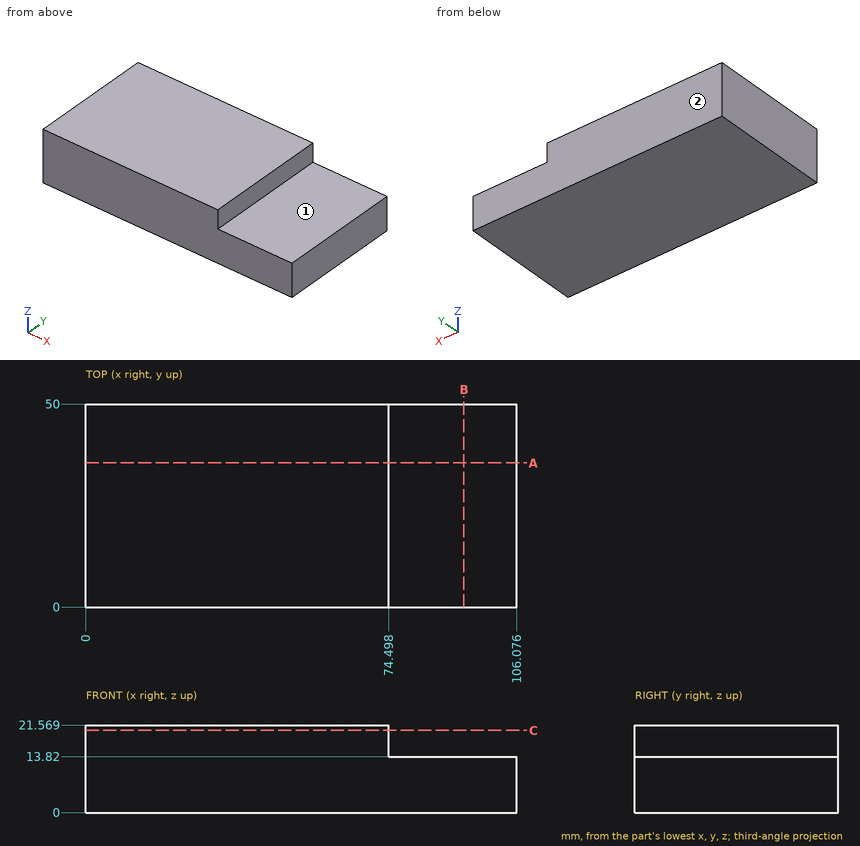
Could you check a few things on this drawing? It's one solid part, dimensions in mm from its lowest x, y, z. A direction names the side the tool comes from. Give positions to 0.01 mm unless a question says otherwise; leave off trailing zeros. Order: outer loops, then holes, each group sorted by start corner. A loop starts at its lowest first (then second) coordinate and runs counter-clockwise, first axis right, second up. Notation, with made-up numbers: (18, 56) -> (40, 56) arc R31 cw to (40, 85) -> close; hole circle Ø2 at (-16.75, 50). An arc over 180 degrees is marked (long way). Use CSV: the item, a comma, the result in double quotes. Start each with the question number.
Item 1: I'm going to push flat-ended pins straight in: P1, Ø2, axis at x = 85, y = 16, coming from the +Z side; P2, Ø4, axis at y = 35, z = 19, coming from the +X side. Where does each tip first touch, or does it pass through?
Item 2: Suppose I cut it at B-B (x = 93). List the corners of the cut face in (y, z) for me.
Item 3: On a 3-axis mill with a long thin cutter (end or side, diameter ignored), from which of +Z, -Z, +X, -X, +Y, -Y can I reach the whole of each face in a straight line? I mean the marked faces 1 and 2. Say none if no direction works.
Item 4: Suppose I cut it at C-C (z = 20.25). List the corners of the cut face in (x, y) for me, and give its area (4 significant figures).
Item 5: Suppose I cut it at A-A (y = 35.5). List the corners of the cut face in (x, z) for me (1 decimal), and give its area (3 significant figures).
Item 6: If I drill on probe 1 along X at (y, z) = (41.5, 20.25); probe 2 along Z at (x, y) = (93.5, 8), over which ranges is the centre line in solid material (lowest first)? Write a range as [from, to].
Answer block:
1,P1,"stops at z = 13.82"
1,P2,"stops at x = 74.5"
2,outline,"(0, 0) -> (50, 0) -> (50, 13.82) -> (0, 13.82) -> close"
3,face 1,"+Z, +X, +Y, -Y"
3,face 2,"+Z, -Z, +X, -X, +Y"
4,outline,"(0, 0) -> (74.5, 0) -> (74.5, 50) -> (0, 50) -> close"
4,area,"3,725 mm^2"
5,outline,"(0, 0) -> (106.1, 0) -> (106.1, 13.8) -> (74.5, 13.8) -> (74.5, 21.6) -> (0, 21.6) -> close"
5,area,"2,040 mm^2"
6,probe 1,"x = [0, 74.5]"
6,probe 2,"z = [0, 13.82]"
